CAD build for the part. Positions are in the model's coordinates, mm. Coordinates: 2 decimals unless noted, no trailing zeros. Order: outer loops, then holes, each group sorted by start corner. A loop starts at its lowest first (then second) coordinate and runs counter-clockwise, first axis right, second up. Notation, with made-up numbers: (64, 81) - (89, 81) arc R21 cw to (89, 95) - close; hole circle Ø11 at (76.5, -27.5). An arc over 180 degrees is marked (long way). Use one line per item in the form item = value.
```python
from build123d import *

# Parameters (mm, degrees)
SKETCH1_R           = 3
BOSS_EXTRUDE2_DEPTH = 2.5


with BuildPart() as part:
    # Sketch1 → Boss-Extrude2 (new, symmetric)
    with BuildSketch(Plane(origin=(0, 0, 0), x_dir=(1, 0, 0), z_dir=(0, 1, 0))):
        Polygon((1.59064416, -6.889836802), (-6.889836802, -1.59064416), (14.185871198, 32.137539077), (76.957416455, 32.137539077), (76.957416455, 22.137539077), (19.728961713, 22.137539077), align=None)
        with Locations(Location((16.957416455, 27.137539077, 0), (0, 0, 270))):
            Circle(SKETCH1_R, mode=Mode.SUBTRACT)
        with Locations(Location((71.957416455, 27.137539077, 0), (0, 0, 270))):
            Circle(SKETCH1_R, mode=Mode.SUBTRACT)
        with Locations(Location((41.957416455, 27.137539077, 0), (0, 0, 270))):
            Circle(SKETCH1_R, mode=Mode.SUBTRACT)
    extrude(amount=BOSS_EXTRUDE2_DEPTH, both=True)


solid = part.part
```
Item 1: Drop flat-ended pins along their axis: pin 1 (1.5 mm diameter, centred on y = 1, z = -2, fed in from -X); pin 2 (2 mm diameter, centred on x = 18, y = 0, fed in from +Z). Give the stop position or say it passes through.
Derived:
pin_1 = -5.11
pin_2 = -17.77
Item 2: Drill centre lines: line 1 (Z direction, x = 61, y = -2.2); line 2 (Z direction, x = 73.5, y = -1.65); line 3 (X direction, y = -2, z = -2.5). Where is each one in solid material? Low to high. Write a range as [from, to].
Derived:
line_1 = [-32.14, -22.14]
line_2 = [-32.14, -29.71], [-24.56, -22.14]
line_3 = [-4.33, 7.46]
Item 3: Cut at C-C, the plane x = 57.5. Write the cut outline in (y, z).
Derived:
outline = (-2.5, -32.14) - (2.5, -32.14) - (2.5, -22.14) - (-2.5, -22.14) - close
Item 4: Two-plate mould, pull along X, no slides. Class faces 1 (the face through (39.03, -0.04, -27.79)), 2 (the face through (49, 0, -22.138)), 3 (the face through (-2.59, 0.035, 4.277)), 4 (the face through (18.985, -0.035, -29.349)): +X half, -X half, draft (parallel to the pull), parting line (faces both ways), or undercut.
Derived:
face_1 = undercut
face_2 = draft
face_3 = -X half
face_4 = undercut
Item 5: Cut at B-B, the plane y = 1.2. Write the cut outline in (x, z).
Derived:
outline = (-6.89, 1.59) - (14.19, -32.14) - (76.96, -32.14) - (76.96, -22.14) - (19.73, -22.14) - (1.59, 6.89) - close; hole circle Ø6 at (16.96, -27.14); hole circle Ø6 at (41.96, -27.14); hole circle Ø6 at (71.96, -27.14)
Item 6: Cut at A-A, the plane x = 70. Write the cut outline in (y, z), plus the area to 3 significant figures.
Derived:
outline = (-2.5, -32.14) - (2.5, -32.14) - (2.5, -29.41) - (-2.5, -29.41) - close; (-2.5, -24.86) - (2.5, -24.86) - (2.5, -22.14) - (-2.5, -22.14) - close
area = 27.3 mm²
Item 7: Cut at D-D, the plane z = -18. Write the cut outline in (x, y).
Derived:
outline = (5.35, -2.5) - (17.14, -2.5) - (17.14, 2.5) - (5.35, 2.5) - close
